Autodesk Inventor part; units mm, degrees
ref_plane "Arbeitsebene1" through (0, 2.5, 0) normal (0, 1, 0) x (-1, 0, 0)
ref_plane "YZ Plane" through (0, 0, 0) normal (1, 0, 0) x (0, 1, 0)
ref_plane "XY Plane" through (0, 0, 0) normal (0, 0, 1) x (1, 0, 0)
sketch "Skizze1" plane through (0, 0, 0) normal (0, 0, 1) x (1, 0, 0)
  circle A0 centre (0, 0) radius 2.5
  dimension "d0" = 5
extrude "Extrusion1" add sketch "Skizze1" along normal blind 50
fillet "Rundung1" radius 2.2 1 edges at (-2.5, 0, 0)
ref_plane "Arbeitsebene1" through (0, 2.5, 0) normal (0, 1, 0) x (-1, 0, 0)
sketch "Skizze2" plane through (0, 2.5, 0) normal (0, 1, 0) x (-1, 0, 0)
  line L0 (2.5, 2.2) -> (2.5, 50)
  line L1 (-2.5, 2.2) -> (-2.5, 50)
  line L2 (2.5, 43.4257) -> (-2.5, 43.4257)
  line L3 (-2.5, 43.4257) -> (-2.5, 37.4257)
  line L4 (-2.5, 37.4257) -> (2.5, 37.4257)
  line L5 (2.5, 37.4257) -> (2.5, 43.4257)
  point P0 (0, 0)
  point P1 (-2.5, 43.4257)
  dimension "d4" = 6
extrude "Extrusion2" cut sketch "Skizze2" against normal blind 0.4
pattern_circular "Runde Anordnung1" count 6 over 360 about axis through (0, 0, -10) along (0, 0, 1) of "Extrusion2"
sketch "Skizze3" plane through (0, 0, 50) normal (0, 0, 1) x (1, 0, 0)
  circle A0 centre (0, 0) radius 2.25
  dimension "d10" = 4.5
extrude "Extrusion3" add sketch "Skizze3" along normal blind 10
properties part number "Thermoelement"
The listing builds one solid part. Answer for the finished solid, in the listing's coordinates (mm). A direction names the side the tool comes from. Give positions to 0.01 mm unless a question says otherwise; leave off trailing zeros. Order: outer loops, then holes, each group sorted by start corner. A loop starts at its lowest first (then second) coordinate and runs counter-clockwise, first axis right, second up. Notation, with made-up numbers: (25.25, 31) -> (40.25, 31) arc R22 ccw to (40.25, 38) -> close; hole circle Ø7 at (23, 13). An arc over 180 degrees is marked (long way). Answer as a JSON object with one key per item and string values. Group by question number.
Item 1: Consider L1, parallel to X at y = -0.2, z = 51; L2, parallel to Y at x = -0.6, z = 40.5; L3, parallel to X at y = 0.25, z = 15.5. Determine where each line is inside the solid, lowest interval first. Write a range as from..to.
Item 2: The part is cut by section A-A on z = 34. Write down the section's boundary in (x, y).
Item 3: Determine the mould class of faces 1 (the flat face through (0, 0, 60)), 2 (the flat face through (-1.81, 1.065, 40.468)), 3 (the cylindrical face through (-0.29, -2.23, 54.93)) for opening direction Z: pulls with the +Z half, pulls with the -Z half, needs draft (parallel to the pull), parting line crosses it, or undercut.
Item 4: A tool of negligible diameter and unlimited length cuts with its end or side. For faces 4 (the flat face through (0, -2.1, 40)), 5 (the flat face through (0, 2.1, 40)), 6 (the flat face through (-1.827, -1.035, 40.468)), 7 (the flat face through (1.827, 1.035, 40.468)), from which of +Z, -Z, +X, -X, +Y, -Y can it reach the whole face along a straight path? Write none if from no direction.
Item 5: Flat-ended cylindrical pins translate along their axes: pin 1 (2.5 mm diameter, centred on x = -0.5, z = 39.5, fed in from -Y); pin 2 (2.5 mm diameter, centred on x = -0.5, z = 40, fed in from +Y). Find the tip coordinate at first contact, or state that the pin passes through.
Result set:
{
 "1": {"L1": "-2.24..2.24", "L2": "-2.1..2.1", "L3": "-2.49..2.49"},
 "2": {"outline": "circle Ø5 at (0, 0)"},
 "3": {"face 1": "pulls with the +Z half", "face 2": "undercut", "face 3": "needs draft"},
 "4": {"face 4": "+X, -X, -Y", "face 5": "+X, -X, +Y", "face 6": "-X, -Y", "face 7": "+X, +Y"},
 "5": {"pin 1": "y = -2.1", "pin 2": "y = 2.1"}
}
